Design review of the part built by this model. Coordinates are the model's own, in mm. Face numbers are marked on the shaded views. A direction names the side the tool comes from. Coordinates: 2 decimals unless noted, no trailing zeros. Order: outer loops, then holes, each group sorted by start corner. A loop starts at its lowest first (then second) coordinate and runs counter-clockwise, first axis right, second up. Notation, with made-up numbers: M 76.5,-35 L 113.5,-35 A12 cw 113.5,-23 Z; hole C 5.25,5.25 d8. An arc over 180 degrees is marked long. Answer in a Markdown table with one row per item.
from build123d import *

# Parameters (mm, degrees)
F1_R     = 20.4097396771
F1_R_2   = 5.0527941738
F2_DEPTH = 5.08
F3_R     = 9.3754452045
F4_DEPTH = 1.524
F6_R     = 1.27


# Not quite as in the source:
# - a feature names something its author has since deleted; it is built from what else it names


with BuildPart() as f2:
    # F1 (on face) → F2 (new body)
    with BuildSketch(Plane.XY):
        Circle(F1_R)
        Circle(F1_R_2, mode=Mode.SUBTRACT)
    extrude(amount=F2_DEPTH)

    # F3 (on Top) → F4 (join)
    with BuildSketch(Plane.XY):
        Circle(F3_R)
    extrude(amount=F4_DEPTH)

    # F6
    f6_edges = [f2.edges().sort_by_distance(p)[0] for p in [
        (-20.40974, 0, 5.08),
    ]]
    fillet(f6_edges, radius=F6_R)


solid = f2.part
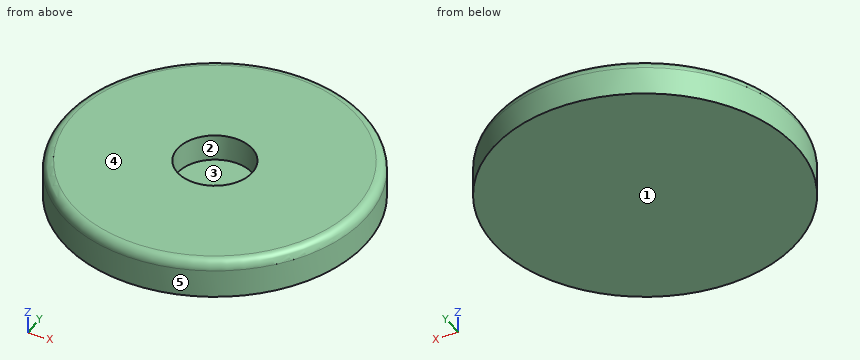
(1) For the marked faces 1 and 2, list the 3-axis set-ups (+Z, -Z, +X, -X, +Y, -Y) from which the entire face can be reached by the end or side of a thin tool; tool diameter is ignored.
Return value:
| item | result |
|---|---|
| face 1 | -Z, +X, -X, +Y, -Y |
| face 2 | +Z |
(2) For line 1 along Y through (x, z) = (0, 3.2); line 2 along X through (y, z) = (-3.5, 2.5); line 3 along Y through (x, z) = (-1.5, 1.75), list the stretches that pass through material, from the lowest coordinate up. Write a range as from..to.
Return value:
| item | result |
|---|---|
| line 1 | y = -20.41..-5.05, 5.05..20.41 |
| line 2 | x = -20.11..-3.64, 3.64..20.11 |
| line 3 | y = -20.35..-4.83, 4.83..20.35 |
(3) Add section A-A, the plane x = 0. Give the boundary of the cut face in (y, z), and give its area (3 significant figures).
Return value:
| item | result |
|---|---|
| outline | M -20.41,0 L 20.41,0 L 20.41,3.81 A1.27 ccw 19.14,5.08 L 5.05,5.08 L 5.05,1.52 L -5.05,1.52 L -5.05,5.08 L -19.14,5.08 A1.27 ccw -20.41,3.81 Z |
| area | 171 mm2 |
(4) Draft analysis for pull direction X (two halves, no side actions). For the marked faces 3, 4 and 5, state which applies: pulls with the +X half, pulls with the -X half, needs draft (parallel to the pull), parting line crosses it, or undercut.
Return value:
| item | result |
|---|---|
| face 3 | undercut |
| face 4 | needs draft |
| face 5 | parting line crosses it |
(5) Insertion check: pin 1 Ø1.5 at (y, z) = (-10.5, 1) entering from +X; pin 2 Ø2 at (x, z) = (9.5, 3.5) entering from +Y. Each pin has a flat end and moves straight along its axis. Give the tip position at first contact, or say it passes through.
Return value:
| item | result |
|---|---|
| pin 1 | stops at x = 17.93 |
| pin 2 | stops at y = 18.56 |
